```python
from build123d import *

# Parameters (mm, degrees)
F0_R     = 11.2014
F1_DEPTH = 7.78
F2_R     = 7.9375
F3_DEPTH = 9.525
F5_D     = 10.1
F6_SIZE2 = 1
F6_SIZE  = 1


with BuildPart() as f1:
    # F0 (on Right) → F1 (new body)
    with BuildSketch(Plane.YZ):
        Circle(F0_R)
    extrude(amount=F1_DEPTH)

    # F2 (on face) → F3 (join)
    with BuildSketch(Plane.YZ.offset(7.78)):
        Circle(F2_R)
    extrude(amount=F3_DEPTH)

    # F5 (through all)
    with Locations(Plane.YZ.offset(17.305)):
        with Locations((0, 0)):
            Hole(F5_D / 2)

    # F6
    f6_edges = [f1.edges().sort_by_distance(p)[0] for p in [
        (17.305, -7.9375, 0),
    ]]
    chamfer(f6_edges, length=F6_SIZE, length2=F6_SIZE2)


solid = f1.part
```
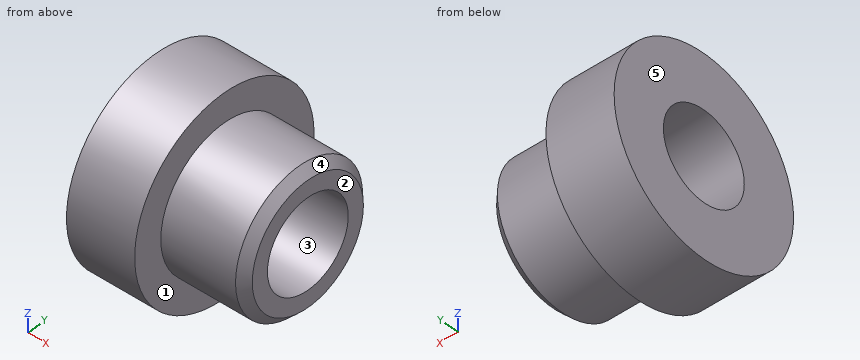
Can you work these out from the model? Positions are in its coordinate system, mm. Face numbers are marked on the shaded views. A direction names the side the tool comes from. Round coordinates to 2 decimals unless told otherwise and drop trailing zeros. Loops run counter-clockwise (first coordinate to the right, second up) from the corner with the lowest first, then second, coordinate; pieces in that order, holes last. Notation, with made-up numbers: (81.5, 69) -> (126.5, 69) arc R13 ccw to (126.5, 85) -> close; hole circle Ø11 at (5, -2). An arc over 180 degrees is marked (long way). Answer in a Markdown table with one row per item.
Item 1: On a 3-axis mill with a long thin cutter (end or side, diameter ignored), from which of +Z, -Z, +X, -X, +Y, -Y can I reach the whole of each face in a straight line? I mean the marked faces 1 and 2. Say none if no direction works.
Answer block:
| item | result |
|---|---|
| face 1 | +X |
| face 2 | +Z, -Z, +X, +Y, -Y |
Item 2: Will these pins go through, and if not, where does the flat tip stop? P1, Ø1, axis at x = 11.5, z = -2.5, coming from the +Y side; P2, Ø9, axis at y = 0, z = 0, coming from the +X side; P3, Ø4, axis at x = 7, y = -5, coming from the +Z side; P4, Ø3, axis at x = 4.5, z = 6.5, coming from the -Y side.
Answer block:
| item | result |
|---|---|
| P1 | y = 7.68 |
| P2 | through |
| P3 | z = 10.79 |
| P4 | y = -10.02 |
Item 3: If I drill on probe 1 along Z at (x, y) = (8, 0); probe 2 along Z at (x, y) = (4.25, 0); probe 3 along X at (y, z) = (2.75, -7.5), over which ranges is the centre line in solid material (lowest first)?
Answer block:
| item | result |
|---|---|
| probe 1 | -7.94 to -5.05, 5.05 to 7.94 |
| probe 2 | -11.2 to -5.05, 5.05 to 11.2 |
| probe 3 | 0 to 7.78 |
Item 4: Suppose I cut it at C-C, the plane x = 3. List the corners of the cut face in (y, z) for me.
Answer block:
| item | result |
|---|---|
| outline | circle Ø22.4 at (0, 0); hole circle Ø10.1 at (0, 0) |
Item 5: We'd pull the mould along Y, two halves only. Please class the marked faces 3, 4 and 5: released by +Y, released by -Y, zero draft, split by the parting line, or undercut.
Answer block:
| item | result |
|---|---|
| face 3 | undercut |
| face 4 | split by the parting line |
| face 5 | zero draft |
